Input: part model. Units: mm. Frame: model coordinates. A direction names the side the tool comes from. Give positions to 0.01 mm unless a question says otherwise; leave off trailing zeros. Loops run counter-clockwise (first coordinate to the right, second up) from the corner with the lowest first, then second, coordinate; pieces in that order, holes last.
from build123d import *

# Parameters (mm, degrees)
SKETCH1_W            = 120
SKETCH1_H            = 175
BOSS_EXTRUDE1_DEPTH  = 2.5
M5_CLEARANCE_HOLE1_D = 5.5
M3_CLEARANCE_HOLE2_D = 3.4
FILLET1_R            = 20
FILLET2_R            = 5
SKETCH11_R           = 2.750000000000002
SKETCH11_R_2         = 1.699999999999985
BOSS_EXTRUDE3_DEPTH  = 5


with BuildPart() as part:
    # Sketch1 → Boss-Extrude1 (new body)
    with BuildSketch(Plane(origin=(0, 0, 0), x_dir=(1, 0, 0), z_dir=(0, 1, 0))):
        Rectangle(SKETCH1_W, SKETCH1_H)
    extrude(amount=BOSS_EXTRUDE1_DEPTH)

    # M5 Clearance Hole1 (through all)
    with Locations(Plane(origin=(0, 2.5, 0), x_dir=(1, 0, 0), z_dir=(0, 1, 0))):
        with Locations((50, 62.5), (50, -2.5), (-20, -77.5), (20, -77.5)):
            Hole(M5_CLEARANCE_HOLE1_D / 2)

    # M3 Clearance Hole2 (through all)
    with Locations(Plane(origin=(0, 2.5, 0), x_dir=(1, 0, 0), z_dir=(0, 1, 0))):
        with Locations((9.76, -59.96), (11.03, -11.7), (-41.04, -44.72), (-41.04, -16.78)):
            Hole(M3_CLEARANCE_HOLE2_D / 2)

    # Fillet1
    fillet1_edges = [part.edges().sort_by_distance(p)[0] for p in [
        (-59.99999999999998, 1.25, -87.50000000000001),
    ]]
    fillet(fillet1_edges, radius=FILLET1_R)

    # Fillet2
    fillet2_edges = [part.edges().sort_by_distance(p)[0] for p in [
        (60.00000000000002, 1.25, 87.49999999999999),
        (-59.99999999999998, 1.25, 87.49999999999999),
        (60.00000000000002, 1.25, -87.50000000000001),
    ]]
    fillet(fillet2_edges, radius=FILLET2_R)

    # Sketch11 → Boss-Extrude3 (add)
    with BuildSketch(Plane(origin=(0, 2.5, 0), x_dir=(1, 0, 0), z_dir=(0, 1, 0))):
        with Locations(Location((-41.039999999999964, -16.779999999999983, 0), (0, 0, 90))):
            Circle(SKETCH11_R)
        with Locations(Location((-41.039999999999964, -16.779999999999983, 0), (0, 0, 270))):
            Circle(SKETCH11_R_2, mode=Mode.SUBTRACT)
    boss_extrude3 = extrude(amount=BOSS_EXTRUDE3_DEPTH)

    # Sketch-Pattern2: Boss-Extrude3 at 3 more places
    with Locations((50.8, 0, 43.18), (52.07, 0, -5.08), (0, 0, 27.94)):
        add(boss_extrude3)


solid = part.part
(1) Pin query (flat end, axial travel): pin 1 Ø4 at (x, z) = (9.76, 59.96) entering from -Y; pin 2 Ø2 at (x, z) = (-28, -44) entering from +Y. Return the tip coordinate at first contact, or that it passes through.
Values follow:
pin 1: stops at y = 0
pin 2: stops at y = 2.5
(2) Cut plane A-A (z = -62.5). Return the cut outline in (x, y), and give its area (3 significant figures).
Values follow:
outline: (-60, 0) - (47.25, 0) - (47.25, 2.5) - (-60, 2.5) - close; (52.75, 0) - (60, 0) - (60, 2.5) - (52.75, 2.5) - close
area: 286 mm2
(3) Ray query, probe 1 along X at (y, z) = (1.5, 77.5); probe 2 along X at (y, z) = (4.15, 11.7); probe 3 along X at (y, z) = (2, 44.72). Return the intervals inside material, ascending.
Values follow:
probe 1: x = -60 to -22.75, -17.25 to 17.25, 22.75 to 60
probe 2: x = 8.28 to 9.33, 12.73 to 13.78
probe 3: x = -60 to -42.74, -39.34 to 60
(4) Cut plane D-D (z = 11.7). Return the cut outline in (x, y), and give its area (3 significant figures).
Values follow:
outline: (-60, 0) - (9.33, 0) - (9.33, 7.5) - (8.28, 7.5) - (8.28, 2.5) - (-60, 2.5) - close; (12.73, 0) - (60, 0) - (60, 2.5) - (13.78, 2.5) - (13.78, 7.5) - (12.73, 7.5) - close
area: 302 mm2
(5) Cut plane C-C (z = 77.5). Return the cut outline in (x, y).
Values follow:
outline: (-60, 0) - (-22.75, 0) - (-22.75, 2.5) - (-60, 2.5) - close; (-17.25, 0) - (17.25, 0) - (17.25, 2.5) - (-17.25, 2.5) - close; (22.75, 0) - (60, 0) - (60, 2.5) - (22.75, 2.5) - close
(6) Mould query, pull axis Z, two halves, no side actions, for faces 3 (the cylindrical face through (-54.297, 1.268, -81.486)), 4 (the flat face through (-39, 7.5, 45)), 5 (the cylindrical face through (-42.899, 4.965, 18.807)). Classes: +Z half, -Z half, draft (parallel to the pull), parting line (faces both ways), or undercut.
Values follow:
face 3: -Z half
face 4: draft
face 5: undercut
(7) Cut plane B-B (y = 4). Return the cut outline in (x, z), and give its area (3 significant figures).
Values follow:
outline: circle Ø5.5 at (-41.04, 16.78); circle Ø5.5 at (-41.04, 44.72); circle Ø5.5 at (9.76, 59.96); circle Ø5.5 at (11.03, 11.7); hole circle Ø3.4 at (-41.04, 16.78); hole circle Ø3.4 at (-41.04, 44.72); hole circle Ø3.4 at (9.76, 59.96); hole circle Ø3.4 at (11.03, 11.7)
area: 58.7 mm2
(8) Reachability of faces 1 (the flat face through (-39, 7.5, 17)), 2 (the cylindrical face through (-41.87, 4.96, 42.1)) from +Z, -Z, +X, -X, +Y, -Y: full face, straight path, thin tool, end or side. Return the list, or none.
Values follow:
face 1: +Z, -Z, +X, -X, +Y
face 2: +Y
